Could you check a few things on this model? Use its own coordinates, in mm. A direction names the side the tool comes from. Round coordinates to 2 decimals unless told otherwise and drop trailing zeros. Loops run counter-clockwise (first coordinate to the right, second up) from the corner with the lowest first, then second, coordinate; pieces in that order, holes last. Notation, with made-up numbers: (25.5, 34) - (60.5, 34) arc R32 ccw to (60.5, 70) - close; hole circle Ø8 at (31, 12.25). An arc over 180 degrees is marked (long way). Use one line per item in the form item = value.
```python
from build123d import *

# Parameters (mm, degrees)
ESBO_O1_R                = 18
ESBO_O1_R_2              = 7.5
RESSALTO_EXTRUS_O1_DEPTH = 24
RESSALTO_EXTRUS_O2_DEPTH = 9
ESBO_O1_4_R              = 12.5
RESSALTO_EXTRUS_O3_DEPTH = 23
ESBO_O1_5_R              = 16
RESSALTO_EXTRUS_O4_DEPTH = 35
ESBO_O2_W                = 34
ESBO_O2_H                = 66.30992931
CORTE_EXTRUS_O1_DEPTH    = 70
ESBO_O3_W                = 48
ESBO_O3_H                = 36
RESSALTO_EXTRUS_O7_DEPTH = 31
ESBO_O4_R                = 7.5
CORTE_EXTRUS_O2_DEPTH    = 48.5


with BuildPart() as part:
    # Esbo_o1 → Ressalto-extrus_o1 (new, symmetric)
    with BuildSketch(Plane(origin=(0, 0, 0), x_dir=(0, 0, -1), z_dir=(1, 0, 0))):
        with Locations((-85, 110)):
            Circle(ESBO_O1_R)
        with Locations((-85, 110)):
            Circle(ESBO_O1_R_2, mode=Mode.SUBTRACT)
    extrude(amount=RESSALTO_EXTRUS_O1_DEPTH, both=True)

    # Esbo_o1_3 → Ressalto-extrus_o2 (add, symmetric)
    with BuildSketch(Plane(origin=(0, 0, 0), x_dir=(0, 0, -1), z_dir=(1, 0, 0))):
        with BuildLine():
            Line((25, 40), (25, 110))
            ThreePointArc((25, 110), (-16.167131291, 90.931075913), (-4.089909266, 134.663183943))
            Line((-4.089909266, 134.663183943), (-85, 128))
            ThreePointArc((-85, 128), (-72.272077939, 122.727922061), (-67, 110))
            ThreePointArc((-67, 110), (-72.272077939, 97.272077939), (-85, 92))
            Line((-85, 92), (-25, 87.058823529))
            Line((-25, 87.058823529), (-25, 40))
            Line((-25, 40), (25, 40))
        make_face()
    extrude(amount=RESSALTO_EXTRUS_O2_DEPTH, both=True)

    # Esbo_o1_4 → Ressalto-extrus_o3 (add, symmetric)
    with BuildSketch(Plane(origin=(0, 0, 0), x_dir=(0, 0, -1), z_dir=(1, 0, 0))):
        with BuildLine():
            ThreePointArc((-4.089909266, 134.663183943), (-16.167131291, 90.931075913), (25, 110))
            ThreePointArc((25, 110), (17.67766953, 127.67766953), (0, 135))
            Line((0, 135), (-4.089909266, 134.663183943))
        make_face()
        with Locations((0, 110)):
            Circle(ESBO_O1_4_R, mode=Mode.SUBTRACT)
    extrude(amount=RESSALTO_EXTRUS_O3_DEPTH, both=True)

    # Esbo_o1_5 → Ressalto-extrus_o4 (add, symmetric)
    with BuildSketch(Plane(origin=(0, 0, 0), x_dir=(0, 0, -1), z_dir=(1, 0, 0))):
        with BuildLine():
            Line((25, 0), (25, 40))
            Line((25, 40), (-25, 40))
            Line((-25, 40), (-25, 0))
            ThreePointArc((-25, 0), (0, -25), (25, 0))
        make_face()
        Circle(ESBO_O1_5_R, mode=Mode.SUBTRACT)
    extrude(amount=RESSALTO_EXTRUS_O4_DEPTH, both=True)

    # Esbo_o2 → Corte-extrus_o1 (cut, symmetric)
    with BuildSketch(Plane.XY):
        with Locations((0, -5.154964655)):
            Rectangle(ESBO_O2_W, ESBO_O2_H)
    extrude(amount=CORTE_EXTRUS_O1_DEPTH, both=True, mode=Mode.SUBTRACT)

    # Esbo_o3 → Ressalto-extrus_o7 (add)
    with BuildSketch(Plane.XY.offset(55)):
        with Locations((0, 110)):
            Rectangle(ESBO_O3_W, ESBO_O3_H)
    extrude(amount=RESSALTO_EXTRUS_O7_DEPTH)

    # Esbo_o4 → Corte-extrus_o2 (cut, symmetric)
    with BuildSketch(Plane(origin=(0, 0, 0), x_dir=(0, 0, -1), z_dir=(1, 0, 0))):
        with Locations((-86, 110)):
            Circle(ESBO_O4_R)
    extrude(amount=CORTE_EXTRUS_O2_DEPTH, both=True, mode=Mode.SUBTRACT)


solid = part.part
```
1. We'd pull the mould along X, two halves only. Please class faces 4 (the face through (23, 121.5, 5.9)), 5 (the face through (10, 128, 70)), 6 (the face through (-17, 13, -11)): +X half, -X half, draft (parallel to the pull), parting line (faces both ways), or undercut.
Solution:
face_4 = +X half
face_5 = draft
face_6 = undercut
2. If we section it at B-B, the plane x = 29.5: Write out the boundary of the cut face in (y, z).
Solution:
outline = (0, -25) - (40, -25) - (40, 25) - (0, 25) arc R25 ccw to start; hole circle Ø32 at (0, 0)
3. If we section it at C-C, the plane z = 68: Write out the boundary of the cut face in (x, y).
Solution:
outline = (-24, 92) - (-9, 92) - (-9, 90.6) - (9, 90.6) - (9, 92) - (24, 92) - (24, 128) - (9, 128) - (9, 129.4) - (-9, 129.4) - (-9, 128) - (-24, 128) - close
4. For P1, Ø1.5, axis at x = -22, y = 41.5, coming from the +Z side; P2, Ø1.5, axis at x = -3, y = 114.5, coming from the -Z side; P3, Ø1.5, axis at x = 26, y = 36, coming from the +Z side; P4, Ø8, axis at x = -21.5, z = 5.5, coming from the +Y side, each with a flat end and sliding along its axis, tell me the tip position at first contact or that it passes through.
Solution:
P1 = through
P2 = -24.72
P3 = 25
P4 = 134.88
5. On a 3-axis mill with a long thin cutter (end or side, diameter ignored), from which of +Z, -Z, +X, -X, +Y, -Y can I reach the whole of each face in a straight line? I mean faces 1 (the face through (-22, 40, 0)), 2 (the face through (-17, 110, 55)), 3 (the face through (10, 92, 70)). Say none if no direction works.
Solution:
face_1 = +Z, -Z, -X
face_2 = -X, +Y, -Y
face_3 = +Z, -Y
6. Please list where these lines run through material, in increasing order: line 1 along Y through (x, z) = (-19.5, -14.5); line 2 along Y through (x, z) = (-5, 86); line 3 along Y through (x, z) = (-28, 0).
Solution:
line_1 = -20.37 to -6.76, 6.76 to 40, 89.63 to 130.37
line_2 = 92.03 to 102.5, 117.5 to 127.97
line_3 = -25 to -16, 16 to 40
7. If we section it at D-D, the plane y = -10.5: Write out the boundary of the cut face in (x, z), plus the area to 3 significant figures.
Solution:
outline = (-35, -22.69) - (-17, -22.69) - (-17, -12.07) - (-35, -12.07) - close; (-35, 12.07) - (-17, 12.07) - (-17, 22.69) - (-35, 22.69) - close; (17, -22.69) - (35, -22.69) - (35, -12.07) - (17, -12.07) - close; (17, 12.07) - (35, 12.07) - (35, 22.69) - (17, 22.69) - close
area = 764 mm^2
8. If we section it at A-A, the plane y = 23: Write out the boundary of the cut face in (x, z), plus the area to 3 significant figures.
Solution:
outline = (-35, -25) - (-17, -25) - (-17, 25) - (-35, 25) - close; (17, -25) - (35, -25) - (35, 25) - (17, 25) - close
area = 1,800 mm^2
